```python
from build123d import *

# Parameters (mm, degrees)
ESQUISSE1_W      = 4.949747468
ESQUISSE1_H      = 4.949747468
EXTRUSION1_DEPTH = 4
EXTRUSION5_DEPTH = 6
CONG_1_R         = 0.5
CONG_2_R         = 0.25


with BuildPart() as part:
    # Esquisse1 → Extrusion1 (new body)
    with BuildSketch(Plane.XY):
        Rectangle(ESQUISSE1_W, ESQUISSE1_H)
    extrude(amount=-EXTRUSION1_DEPTH)

    # Esquisse3 → Extrusion5 (add)
    with BuildSketch(Plane.XY):
        with BuildLine():
            Line((-1.322875656, 1.5), (1.322875656, 1.5))
            ThreePointArc((1.322875656, 1.5), (2, 0), (1.322875656, -1.5))
            Line((1.322875656, -1.5), (-1.322875656, -1.5))
            ThreePointArc((-1.322875656, -1.5), (-2, 0), (-1.322875656, 1.5))
        make_face()
    extrude(amount=EXTRUSION5_DEPTH)

    # Congé1
    cong_1_edges = [part.edges().sort_by_distance(p)[0] for p in [
        (2.474873734, 0, -4),
        (0, 2.474873734, -4),
        (-2.474873734, 0, -4),
        (0, -2.474873734, -4),
        (-2.474873734, 2.474873734, -2),
        (2.474873734, 2.474873734, -2),
        (2.474873734, -2.474873734, -2),
        (-2.474873734, -2.474873734, -2),
    ]]
    fillet(cong_1_edges, radius=CONG_1_R)

    # Congé2
    cong_2_edges = [part.edges().sort_by_distance(p)[0] for p in [
        (-2, 0, 6),
        (0, -1.5, 6),
        (2, 0, 6),
        (0, 1.5, 6),
    ]]
    fillet(cong_2_edges, radius=CONG_2_R)


solid = part.part
```
Build history of the part. All positions in model axes, mm. A direction names the side the tool comes from. Coordinates: 2 decimals unless noted, no trailing zeros. Order: outer loops, then holes, each group sorted by start corner. A loop starts at its lowest first (then second) coordinate and runs counter-clockwise, first axis right, second up. Notation, with made-up numbers: (-23.75, -23) -> (-17.75, -23) arc R30 ccw to (-17.75, 10) -> close; hole circle Ø3 at (23, 86.25). An arc over 180 degrees is marked (long way). Answer in a Markdown table with one row per item. Add a question column.
Q1. Which spindle directions (+Z, -Z, +X, -X, +Y, -Y) get a long thin tool onto all of the face, cutting with end or side? Do faces 1 (the face through (0, 1.5, 3)), 2 (the face through (-2, 0, 3)), 3 (the face through (2, 0, 3)), 4 (the face through (0, -1.5, 3)), 5 (the face through (0, 2.475, -2)). Say none if no direction does.
Q2. Wall check: line 1 along Y through (x, z) = (0.1, 1.75); line 2 along Z through (x, y) = (-0.3, -1.55); line 3 along X through (y, z) = (-2.15, -2). Give the ranges that are in metal, low to high. Write a range as [from, to].
Q3. Band-saw the part on B-B, the plane z = 5.25. List the corners of the cut face in (x, y).
Q4. Drop flat-ended pins along their axis: pin 1 (0.8 mm diameter, centred on x = -0.5, z = 3.5, fed in from +Y); pin 2 (2 mm diameter, centred on x = 0, z = 3, fed in from -Y). Give the stop position or say it passes through.
Q5. Band-saw the part on A-A, the plane x = -0.1. List the corners of the cut face in (y, z).
Answers follow:
| question | item | result |
|---|---|---|
| 1 | face 1 | +Z, +X, -X, +Y |
| 1 | face 2 | +Z, -X |
| 1 | face 3 | +Z, +X |
| 1 | face 4 | +Z, +X, -X, -Y |
| 1 | face 5 | +Z, -Z, +X, -X, +Y |
| 2 | line 1 | [-1.5, 1.5] |
| 2 | line 2 | [-4, 0] |
| 2 | line 3 | [-2.44, 2.44] |
| 3 | outline | (-1.32, -1.5) -> (1.32, -1.5) arc R2 ccw to (1.32, 1.5) -> (-1.32, 1.5) arc R2 ccw to start |
| 4 | pin 1 | y = 1.5 |
| 4 | pin 2 | y = -1.5 |
| 5 | outline | (-2.47, -3.5) arc R0.5 ccw to (-1.97, -4) -> (1.97, -4) arc R0.5 ccw to (2.47, -3.5) -> (2.47, 0) -> (1.5, 0) -> (1.5, 5.75) arc R0.25 ccw to (1.25, 6) -> (-1.25, 6) arc R0.25 ccw to (-1.5, 5.75) -> (-1.5, 0) -> (-2.47, 0) -> close |
